```python
from build123d import *

# Parameters (mm, degrees)
SKETCH1_W           = 56
SKETCH1_H           = 48
SKETCH1_R           = 1.65
SKETCH1_W_2         = 36
SKETCH1_H_2         = 36
BOSS_EXTRUDE1_DEPTH = 2
FILLET1_R           = 1.6


with BuildPart() as part:
    # Sketch1 → Boss-Extrude1 (new body)
    with BuildSketch(Plane(origin=(0, 0, 0), x_dir=(1, 0, 0), z_dir=(0, 1, 0))):
        Rectangle(SKETCH1_W, SKETCH1_H)
        with Locations((-24, 20)):
            Circle(SKETCH1_R, mode=Mode.SUBTRACT)
        with Locations((-24, -20)):
            Circle(SKETCH1_R, mode=Mode.SUBTRACT)
        with Locations((24, 20)):
            Circle(SKETCH1_R, mode=Mode.SUBTRACT)
        with Locations((24, -20)):
            Circle(SKETCH1_R, mode=Mode.SUBTRACT)
        Rectangle(SKETCH1_W_2, SKETCH1_H_2, mode=Mode.SUBTRACT)
    extrude(amount=BOSS_EXTRUDE1_DEPTH)

    # Fillet1
    fillet1_edges = [part.edges().sort_by_distance(p)[0] for p in [
        (18, 1, -18),
        (-18, 1, -18),
        (-18, 1, 18),
        (18, 1, 18),
    ]]
    fillet(fillet1_edges, radius=FILLET1_R)


solid = part.part
```
The model under review builds one solid part; all positions refer to its coordinate system, in mm. A direction names the side the tool comes from. Give positions to 0.01 mm unless a question says otherwise; leave off trailing zeros. Write each loop counter-clockwise with the first axis right and the second up, starting at its lowest first coordinate (ties: lowest second). Pieces come first, ordered by that corner, then holes. Notation, with made-up numbers: (22, 77) - (50, 77) arc R10 ccw to (50, 93) - close; hole circle Ø11 at (-29, 88). An arc over 180 degrees is marked (long way). Answer in a Markdown table with one row per item. Add a question column.
1. Tool access review of faces 1 (the flat face through (28, 1, 0)), 2 (the cylindrical face through (-17.52, 1.01, -17.54)): name each direction out of +Z, -Z, +X, -X, +Y, -Y from which nothing blocks a thin tool from reaching the whole face with its end or side.
2. Draft analysis for pull direction X (two halves, no side actions). For faces 3 (the cylindrical face through (-17.52, 1.01, 17.54)), 4 (the flat face through (-19, 0, 0)), 5 (the cylindrical face through (22.784, 0.986, 18.885)), 6 (the flat face through (-28, 1, 0)), state which applies: +X half, -X half, draft (parallel to the pull), parting line (faces both ways), or undercut.
3. We need section C-C on y = 0.8. Write out the cut boundary in (x, z), then the cut area to 3 significant figures.
4. We need section A-A on z = 14. Write out the cut boundary in (x, y).
5. We need section D-D on z = -20. Write out the cut boundary in (x, y), then the cut area to 3 significant figures.
6. Insertion check: P1, Ø4, axis at x = 24, z = -20, coming from the +Y side. The pin has a flat end and moves straight along its axis. Give the tip position at first contact, or say it passes through.
7. Wall thickness on line 1 along Z through (x, y) = (-24, 1.5); line 2 along X through (y, z) = (0.7, 20); line 3 along Z through (x, y) = (6.5, 1.1): over which ranges is each line inside the solid? List them lowest first. Write a range as [from, to].
8. We need section B-B on x = 24. Write out the cut boundary in (y, z), then the cut area to 3 significant figures.
Ans:
| question | item | result |
|---|---|---|
| 1 | face 1 | +Z, -Z, +X, +Y, -Y |
| 1 | face 2 | +Y, -Y |
| 2 | face 3 | undercut |
| 2 | face 4 | draft |
| 2 | face 5 | undercut |
| 2 | face 6 | -X half |
| 3 | outline | (-28, -24) - (28, -24) - (28, 24) - (-28, 24) - close; hole circle Ø3.3 at (-24, -20); hole circle Ø3.3 at (-24, 20); hole (-18, -16.4) arc R1.6 ccw to (-16.4, -18) - (16.4, -18) arc R1.6 ccw to (18, -16.4) - (18, 16.4) arc R1.6 ccw to (16.4, 18) - (-16.4, 18) arc R1.6 ccw to (-18, 16.4) - close; hole circle Ø3.3 at (24, -20); hole circle Ø3.3 at (24, 20) |
| 3 | area | 1,360 mm^2 |
| 4 | outline | (-28, 0) - (-18, 0) - (-18, 2) - (-28, 2) - close; (18, 0) - (28, 0) - (28, 2) - (18, 2) - close |
| 5 | outline | (-28, 0) - (-25.65, 0) - (-25.65, 2) - (-28, 2) - close; (-22.35, 0) - (22.35, 0) - (22.35, 2) - (-22.35, 2) - close; (25.65, 0) - (28, 0) - (28, 2) - (25.65, 2) - close |
| 5 | area | 98.8 mm^2 |
| 6 | P1 | stops at y = 2 |
| 7 | line 1 | z = [-24, -21.65], [-18.35, 18.35], [21.65, 24] |
| 7 | line 2 | x = [-28, -25.65], [-22.35, 22.35], [25.65, 28] |
| 7 | line 3 | z = [-24, -18], [18, 24] |
| 8 | outline | (0, -24) - (2, -24) - (2, -21.65) - (0, -21.65) - close; (0, -18.35) - (2, -18.35) - (2, 18.35) - (0, 18.35) - close; (0, 21.65) - (2, 21.65) - (2, 24) - (0, 24) - close |
| 8 | area | 82.8 mm^2 |
